Check sheet for the modelled part. Datum: model origin and axes. Units: mm. Coordinates: 2 decimals unless noted, no trailing zeros. Write each loop counter-clockwise with the first axis right and the second up, starting at its lowest first coordinate (ties: lowest second). Pieces come first, ordered by that corner, then holes. Notation, with made-up numbers: M -27,-1 L 15,-1 A10 ccw 15,7 Z; hole C 39.5,2 d4. An arc over 180 degrees is marked long. Answer as CSV lines item,"result". Start each with the question number.
Q1. Depth check by flat-ended pin: pin 1 Ø1 at (x, y) = (11.5, -2.5) entering from +Z; pin 2 Ø6 at (y, z) = (-1, 2.5) entering from -X; pin 3 Ø2 at (x, z) = (4.5, 2.5) entering from +Y. Enter the tip coordinate at first touch or a pass-through.
Q2. Sectioned sample at A-A, the plane x = 5. Record the cut outline in (y, z), then the cut area to 3 significant figures.
Q3. Mould release check, pull along X, two halves, no side actions. Record for faces 1 (the cylindrical face through (14.8, -1.08, 4.88)), 2 (the flat face through (30, 0, 0)), 3 (the flat face through (0, 0, 0)): pulls with the +X half, pulls with the -X half, needs draft (parallel to the pull), parting line crosses it, or undercut.
Q4. Thickness scan on line 1 along Z through (x, y) = (14.5, -2.5); line 2 along X through (y, z) = (-2.25, -3.75); line 3 along X through (y, z) = (2.75, -3.5). Record the ranges inside material, lowest first. Write a range as from..to.
Autodesk Inventor part; units mm, degrees
ref_plane "YZ Plane" through (0, 0, 0) normal (1, 0, 0) x (0, 1, 0)
ref_plane "XZ Plane" through (0, 0, 0) normal (0, 1, 0) x (-1, 0, 0)
ref_plane "XY Plane" through (0, 0, 0) normal (0, 0, 1) x (1, 0, 0)
sketch "Skizze" plane through (0, 0, 0) normal (1, 0, 0) x (0, 1, 0)
  circle A0 centre (0, 0) radius 5
  dimension "d1" = 10
extrude "Körper" add sketch "Skizze" along normal blind 30
chamfer "Fase1" distance 1 angle 45 1 edges at (0, -5, 0) measured on face at (20, 4.9838, -0.4023)
chamfer "Skizze2" distance 1 angle 45 1 edges at (30, -5, 0) measured on face at (20.3333, 4.9838, -0.4023)
equation "\"d1\" = NND"
equation "\"d2\" = NLG"
equation "\"d4\" = PHH"
equation "\"d5\" = FAWI"
equation "\"d11\" = PHH"
equation "\"d8\" = PHH"
equation "\"d9\" = FAWI"
equation "\"d12\" = PHH"
equation "\"NND\" = 10"
equation "\"NLG\" = 30"
equation "\"PHH\" = 1"
equation "\"FAWI\" = 45deg"
equation "\"KAH\" = 0.8"
equation "\"NLG1\" = 32"
properties part number "CNS 397 - 10 x 30" material "Stahl, weich"
Output:
1,pin 1,"stops at z = 4.58"
1,pin 2,"stops at x = 0"
1,pin 3,"stops at y = 4.77"
2,outline,"C 0,0 d10"
2,area,"78.5 mm^2"
3,face 1,"needs draft"
3,face 2,"pulls with the +X half"
3,face 3,"pulls with the -X half"
4,line 1,"z = -4.33..4.33"
4,line 2,"x = 0.37..29.63"
4,line 3,"x = 0.45..29.55"
